CAD build for the part. Positions are in the model's coordinates, mm. Give positions to 0.01 mm unless a question says otherwise; leave off trailing zeros. Write each loop counter-clockwise with the first axis right and the second up, starting at its lowest first coordinate (ties: lowest second). Pieces come first, ordered by that corner, then holes. Notation, with made-up numbers: (34.5, 33.5) - (71.5, 33.5) arc R10 ccw to (71.5, 44.5) - close; hole circle Ø5 at (74.25, -32). An arc over 180 degrees is marked (long way). Answer as a JSON object with one key per item and string values.
from build123d import *

# Parameters (mm, degrees)
SKETCH1_W                 = 6.35
SKETCH1_H                 = 19.05
EXTRUDE1_DEPTH            = 114.3
M6X1_0_TAPPED_HOLE1_D     = 5
M6X1_0_TAPPED_HOLE1_DEPTH = 6.35


with BuildPart() as part:
    # Sketch1 → Extrude1 (new body, symmetric)
    with BuildSketch(Plane.XY):
        Rectangle(SKETCH1_W, SKETCH1_H)
    extrude(amount=EXTRUDE1_DEPTH, both=True)

    # M6x1.0 Tapped Hole1
    with Locations(Plane(origin=(3.175, 0, 0), x_dir=(0, 0, -1), z_dir=(1, 0, 0))):
        with Locations((-101.6, 0), (101.6, 0)):
            Hole(M6X1_0_TAPPED_HOLE1_D / 2, depth=M6X1_0_TAPPED_HOLE1_DEPTH)


solid = part.part
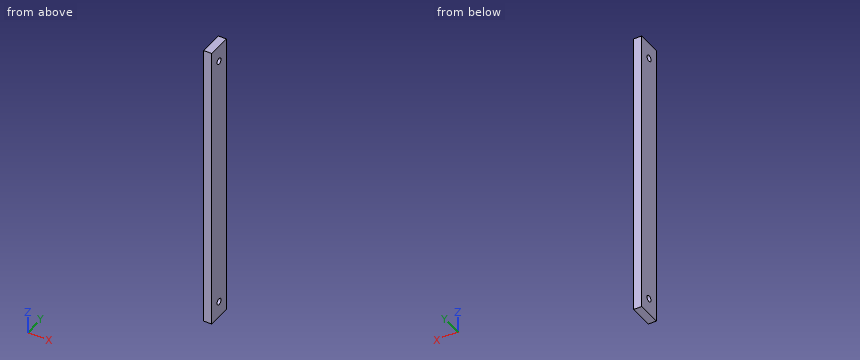
(1) Flat gauge pin, fed straight in: P1, Ø6, axis at y = 0, z = 101.6, coming from the +X side (3 decimals). Where does the tip first touch, or does it go through?
Answer key:
{"P1": "stops at x = 3.175"}
(2) Saw through at B-B, the plane z = 101.6. Give the cut face in (x, y) (3 decimals).
Answer key:
{"outline": "(-3.175, -9.525) - (3.175, -9.525) - (3.175, -2.5) - (-3.175, -2.5) - close; (-3.175, 2.5) - (3.175, 2.5) - (3.175, 9.525) - (-3.175, 9.525) - close"}
(3) Probe L1, parallel to Y at x = -0.25, z = -101.6 (3 decimals); L2, parallel to Z at x = 2.5, y = 2. List the from-to ranges inside material, lowest first. Write a range as [from, to].
Answer key:
{"L1": "y = [-9.525, -2.5], [2.5, 9.525]", "L2": "z = [-114.3, -103.1], [-100.1, 100.1], [103.1, 114.3]"}
(4) Saw through at A-A, the plane y = 0. Give the cut face in (x, z) (3 decimals), and give its area (3 significant figures).
Answer key:
{"outline": "(-3.175, -114.3) - (3.175, -114.3) - (3.175, -104.1) - (-3.175, -104.1) - close; (-3.175, -99.1) - (3.175, -99.1) - (3.175, 99.1) - (-3.175, 99.1) - close; (-3.175, 104.1) - (3.175, 104.1) - (3.175, 114.3) - (-3.175, 114.3) - close", "area": "1,390 mm²"}
